```python
from build123d import *

# Parameters (mm, degrees)
BOSS_EXTRUDE2_DEPTH = 25.4
SKETCH2_R           = 3.2639
CUT_EXTRUDE1_DEPTH  = 71.138042459


with BuildPart() as part:
    # Sketch1 → Boss-Extrude2 (new body)
    with BuildSketch(Plane.XY):
        with BuildLine():
            Line((50.8, 0), (57.15, 0))
            Line((57.15, 0), (57.15, 29.21))
            ThreePointArc((57.15, 29.21), (56.406051224, 31.006051224), (54.61, 31.75))
            Line((54.61, 31.75), (-6.35, 31.75))
            ThreePointArc((-6.35, 31.75), (-19.678174928, 26.028174928), (-25.4, 12.7))
            Line((-25.4, 12.7), (-25.4, 0))
            Line((-25.4, 0), (0, 0))
            Line((0, 0), (0, 25.4))
            Line((0, 25.4), (50.8, 25.4))
            Line((50.8, 25.4), (50.8, 0))
        make_face()
        Polygon((-8.489396689, 4.967655623), (-4.955326016, 11.392114963), (-8.752035673, 17.664939614), (-16.082816004, 17.513304926), (-19.616886677, 11.088845586), (-15.820177019, 4.816020934), align=None, mode=Mode.SUBTRACT)
    extrude(amount=BOSS_EXTRUDE2_DEPTH)

    # Sketch2 → Cut-Extrude1 (cut, through all)
    with BuildSketch(Plane(origin=(0, 31.75, 0), x_dir=(1, 0, 0), z_dir=(0, 1, 0))):
        with Locations(Location((12.7, -12.7, 0), (0, 0, 180))):
            Circle(SKETCH2_R)
        with Locations(Location((38.1, -12.7, 0), (0, 0, 270))):
            Circle(SKETCH2_R)
    extrude(amount=-CUT_EXTRUDE1_DEPTH, mode=Mode.SUBTRACT)


solid = part.part
```
Can you work these out from the model? Positions are in its coordinate system, mm. A direction names the side the tool comes from. Coordinates: 2 decimals unless noted, no trailing zeros. Write each loop counter-clockwise with the first axis right and the second up, starting at its lowest first coordinate (ties: lowest second). Pieces come first, ordered by that corner, then holes. Notation, with made-up numbers: M -35.5,59.5 L -11.5,59.5 A36 ccw -11.5,95.5 Z; hole C 25.5,-16.75 d5. An arc over 180 degrees is marked long. Answer as CSV lines item,"result".
Item 1: Imagine slicing it at A-A on y = 4. List the corners of the cut face in (x, z) for me.
Geometry results:
outline,"M -25.4,0 L 0,0 L 0,25.4 L -25.4,25.4 Z; M 50.8,0 L 57.15,0 L 57.15,25.4 L 50.8,25.4 Z"
Item 2: I'm going to push flat-ended pins straight in: P1, Ø7.5, axis at x = 15.5, z = 12.5, coming from the -Y side; P2, Ø3, axis at y = 21.5, z = 20, coming from the -X side. Where does each tip first touch, or does it pass through?
Geometry results:
P1,"stops at y = 25.4"
P2,"stops at x = -23.78"
Item 3: Please list where these lines run through material, in increasing order: line 1 along X through (y, z) = (6, 11.5); line 2 along Z through (x, y) = (12.7, 27); line 3 along X through (y, z) = (9, 3.5).
Geometry results:
line 1,"x = -25.4 to -16.54, -7.92 to 0, 50.8 to 57.15"
line 2,"z = 0 to 9.44, 15.96 to 25.4"
line 3,"x = -25.4 to -18.35, -6.27 to 0, 50.8 to 57.15"
Item 4: We'd pull the mould along Y, two halves only. Please class faces 1 (the flat face through (-6.75, 8.13, 12.52)), 2 (the flat face through (-13, 0, 13)), 3 (the flat face through (-17.745, 7.996, 12.522)), 4 (the flat face through (25, 31.75, 13)): +Y half, -Y half, draft (parallel to the pull), parting line (faces both ways), or undercut.
Geometry results:
face 1,"undercut"
face 2,"-Y half"
face 3,"undercut"
face 4,"+Y half"
Item 5: On a 3-axis mill with a long thin cutter (end or side, diameter ignored), from which of +Z, -Z, +X, -X, +Y, -Y can I reach the whole of each face in a straight line? I mean faces 5 (the flat face through (50.8, 13, 13)), 6 (the flat face through (-17.825, 14.346, 12.522)), 7 (the flat face through (15, 27, 0)). Say none if no direction works.
Geometry results:
face 5,"+Z, -Z, -Y"
face 6,"+Z, -Z"
face 7,"-Z, +X, -X, +Y, -Y"
Item 6: Imagine slicing it at C-C on x = 38.1. List the corners of the cut face in (y, z) for me, plus the area to 3 significant figures.
Geometry results:
outline,"M 25.4,0 L 31.75,0 L 31.75,9.44 L 25.4,9.44 Z; M 25.4,15.96 L 31.75,15.96 L 31.75,25.4 L 25.4,25.4 Z"
area,"120 mm2"
Item 7: Imagine slicing it at B-B on z = 12.7. List the corners of the cut face in (x, y) for me, plus the area to 3 significant figures.
Geometry results:
outline,"M -25.4,0 L 0,0 L 0,25.4 L 9.44,25.4 L 9.44,31.75 L -6.35,31.75 A19.56 ccw -25.4,12.7 Z; M 15.96,25.4 L 34.84,25.4 L 34.84,31.75 L 15.96,31.75 Z; M 41.36,25.4 L 50.8,25.4 L 50.8,0 L 57.15,0 L 57.15,29.21 A2.54 ccw 54.61,31.75 L 41.36,31.75 Z; hole M -19.62,11.09 L -15.82,4.82 L -8.49,4.97 L -4.96,11.39 L -8.75,17.66 L -16.08,17.51 Z"
area,"1,020 mm2"
Item 8: Imagine slicing it at D-D on z = 20. List the corners of the cut face in (x, y) for me, plus the area to 3 significant figures.
Geometry results:
outline,"M -25.4,0 L 0,0 L 0,25.4 L 50.8,25.4 L 50.8,0 L 57.15,0 L 57.15,29.21 A2.54 ccw 54.61,31.75 L -6.35,31.75 A19.56 ccw -25.4,12.7 Z; hole M -19.62,11.09 L -15.82,4.82 L -8.49,4.97 L -4.96,11.39 L -8.75,17.66 L -16.08,17.51 Z"
area,"1,110 mm2"
